Part model, mm, in its own coordinate system. Round coordinates to 2 decimals unless told otherwise and drop trailing zeros. Write each loop counter-clockwise with the first axis right and the second up, starting at its lowest first coordinate (ties: lowest second). Pieces come first, ordered by that corner, then holes.
1) Saw through at C-C on y = -15. Write the cut outline in (x, z), and give its area (3 significant figures).
2) Drill centre lines: L1, parallel to X at y = 4.5, z = -2.5; L2, parallel to Y at x = -0.3, z = -0.75; L3, parallel to Z at x = 0.5, y = -6. Where is each one in solid material? Low to high.
3) Flat gauge pins, fed straight in: pin 1 (1.1 mm diameter, centred on x = 1.5, z = 0, fed in from +Y); pin 2 (3 mm diameter, centred on y = -14.57, z = 0, fed in from +X); pin 3 (0.8 mm diameter, centred on x = 1.5, y = 0, fed in from +Z); pin 4 (2.5 mm diameter, centred on y = 14.87, z = 0, fed in from -X). Where does each tip first touch, or does it go through?
4) Saw through at D-D on y = 0. Write the cut outline in (x, z), and give its area (3 significant figures).
5) Saw through at B-B on x = -0.4. Write the cut outline in (y, z), and give its area (3 significant figures).
6) Saw through at A-A on z = 0. Write the cut outline in (x, y), and give its area (3 significant figures).
```python
from build123d import *

# Parameters (mm, degrees)
F0_R     = 0.9906
F0_R_2   = 1.5494
F1_DEPTH = 0.7366
F2_W     = 3.4925
F2_H     = 1.905
F3_DEPTH = 1.016
F5_DEPTH = 25.4


with BuildPart() as f1:
    # F0 (on Right) → F1 (new body, symmetric)
    with BuildSketch(Plane.YZ):
        Polygon((19.9517, 3.0861), (-3.0353, 3.0861), (-3.0353, 1.8161), (-19.9517, 1.8161), (-19.9517, -1.8923), (-15.9893, -1.8923), (-15.9893, -3.0861), (19.9517, -3.0861), align=None)
        with Locations((-14.5669, 0)):
            Circle(F0_R, mode=Mode.SUBTRACT)
        with Locations((14.8717, 0)):
            Circle(F0_R_2, mode=Mode.SUBTRACT)
    extrude(amount=F1_DEPTH, both=True)

    # F2 (on face) → F3 (join)
    with BuildSketch(Plane.YZ.offset(0.7366)):
        with Locations((-0.00635, 0)):
            Rectangle(F2_W, F2_H)
    extrude(amount=F3_DEPTH)

    # F4 (on face) → F5 (cut)
    with BuildSketch(Plane(origin=(0, 0, -0.9525), x_dir=(1, 0, 0), z_dir=(0, 0, -1))):
        Polygon((1.7526, 1.7526), (0.7366, 1.7526), (1.7526, -1.7399), align=None)
    extrude(amount=-F5_DEPTH, mode=Mode.SUBTRACT)


solid = f1.part
```
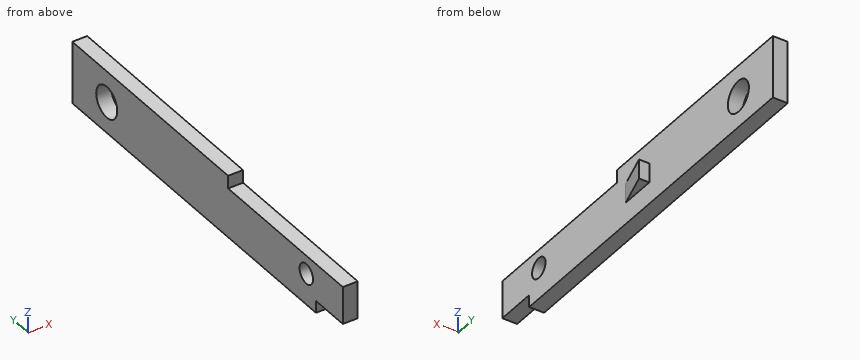
Completed:
1. outline: (-0.74, -3.09) - (0.74, -3.09) - (0.74, -0.89) - (-0.74, -0.89) - close; (-0.74, 0.89) - (0.74, 0.89) - (0.74, 1.82) - (-0.74, 1.82) - close
1. area: 4.60 mm2
2. L1: x = -0.74 to 0.74
2. L2: y = -19.95 to -15.21, -13.92 to 13.52, 16.23 to 19.95
2. L3: z = -3.09 to 1.82
3. pin 1: stops at y = 1.74
3. pin 2: stops at x = 0.74
3. pin 3: stops at z = 0.95
3. pin 4: passes through
4. outline: (-0.74, -3.09) - (0.74, -3.09) - (0.74, -0.95) - (1.25, -0.95) - (1.25, 0.95) - (0.74, 0.95) - (0.74, 3.09) - (-0.74, 3.09) - close
4. area: 10.1 mm2
5. outline: (-19.95, -1.89) - (-15.99, -1.89) - (-15.99, -3.09) - (19.95, -3.09) - (19.95, 3.09) - (-3.04, 3.09) - (-3.04, 1.82) - (-19.95, 1.82) - close; hole circle Ø1.98 at (-14.57, 0); hole circle Ø3.1 at (14.87, 0)
5. area: 209 mm2
6. outline: (-0.74, -19.95) - (0.74, -19.95) - (0.74, -15.56) - (-0.74, -15.56) - close; (-0.74, -13.58) - (0.74, -13.58) - (0.74, -1.75) - (1.75, 1.74) - (0.74, 1.74) - (0.74, 13.32) - (-0.74, 13.32) - close; (-0.74, 16.42) - (0.74, 16.42) - (0.74, 19.95) - (-0.74, 19.95) - close
6. area: 53.1 mm2
